The model under review builds one solid part; all positions refer to its coordinate system, in mm. Face numbers are marked on the shaded views. A direction names the side the tool comes from. Give positions to 0.01 mm unless a question says otherwise; leave off trailing zeros. Order: outer loops, then holes, each group sorted by start corner. A loop starts at its lowest first (then second) coordinate and runs counter-clockwise, first axis right, second up. Notation, with made-up numbers: (-19.75, 85) - (38.25, 85) arc R17 cw to (38.25, 99) - close; hole circle Ø6 at (-38.5, 12.5). An arc over 180 degrees is marked (long way). Use a Markdown table: item, result. Add a question column.
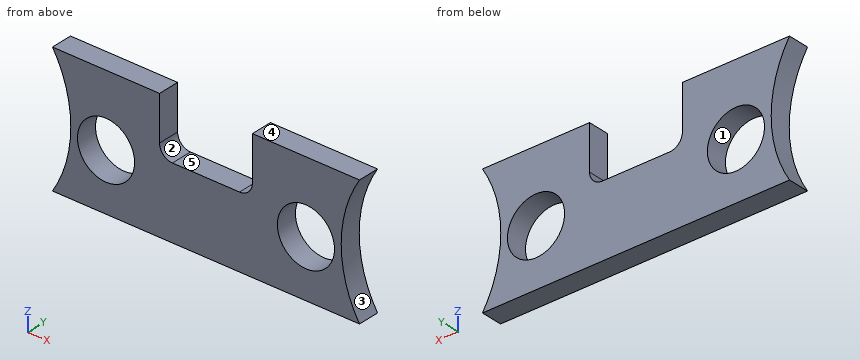
```python
from build123d import *

# Parameters (mm, degrees)
F0_W     = 273.05
F0_H     = 114.3
F1_DEPTH = 19.05
F2_R     = 25.4
F3_DEPTH = 25.4
F5_DEPTH = 25.4
F7_DEPTH = 25.4


with BuildPart() as f1:
    # F0 (on Front) → F1 (new body)
    with BuildSketch(Plane.XZ):
        with Locations((136.525, 57.15)):
            Rectangle(F0_W, F0_H)
    extrude(amount=F1_DEPTH)

    # F2 (on face) → F3 (cut)
    with BuildSketch(Plane.XZ.offset(19.05)):
        with Locations((47.625, 50.8)):
            Circle(F2_R)
        with Locations((225.425, 50.8)):
            Circle(F2_R)
    extrude(amount=-F3_DEPTH, mode=Mode.SUBTRACT)

    # F4 (on face) → F5 (cut)
    with BuildSketch(Plane.XZ.offset(19.05)):
        with BuildLine():
            Line((177.8, 114.3), (95.25, 114.3))
            Line((95.25, 114.3), (95.25, 74.93))
            ThreePointArc((95.25, 74.93), (98.597769, 66.847769), (106.68, 63.5))
            Line((106.68, 63.5), (166.37, 63.5))
            ThreePointArc((166.37, 63.5), (174.452231, 66.847769), (177.8, 74.93))
            Line((177.8, 74.93), (177.8, 114.3))
        make_face()
    extrude(amount=-F5_DEPTH, mode=Mode.SUBTRACT)

    # F6 (on face) → F7 (cut)
    with BuildSketch(Plane.XZ.offset(19.05)):
        with BuildLine():
            Line((0, 114.3), (0, 0))
            ThreePointArc((0, 0), (16.273098, 57.15), (0, 114.3))
        make_face()
        with BuildLine():
            ThreePointArc((273.05, 114.3), (256.776902, 57.15), (273.05, 0))
            Line((273.05, 0), (273.05, 114.3))
        make_face()
    extrude(amount=-F7_DEPTH, mode=Mode.SUBTRACT)


solid = f1.part
```
Q1. Wall thickness on probe 1 along X at (y, z) = (-2.5, 48); probe 2 along X at (y, z) = (-9.25, 62); probe 3 along Z at (x, y) = (161, -14): over which ranges is each line inside the solid? List them lowest first.
Q2. We need section B-B (z = 93). Write out the cut boundary in (x, y), plus the area to 3 significant figures.
Q3. Draft analysis for pull direction X (two halves, no side actions). For the marked faces 3, 4 and 5, state which applies: pulls with the +X half, pulls with the -X half, needs draft (parallel to the pull), parting line crosses it, or undercut.
Q4. Machinability: for the marked faces 1 and 2, which of the approach directions +Z, -Z, +X, -X, +Y, -Y give a long, thin tool a straight path to every point of the face, cutting with its end or side? Answer none if there is none.
Q5. We need section C-C (x = 31). Write out the cut boundary in (y, z), plus the area to 3 significant figures.
Q6. Clearance check with flat-ended pins moving along their axes: P1, Ø6, axis at x = 114, y = -9.5, coming from the +Z side; P2, Ø2, axis at y = -13, z = 55.5, coming from the -X side; P3, Ø2, axis at y = -8.5, z = 91.5, coming from the -X side. State where each tip first meets the part, or that it passes through.
Q7. We need section D-D (z = 50.8). Write out the cut boundary in (x, y) (3 decimals), plus the area to 3 significant figures.
Q8. We need section A-A (y = -10.5). Write out the cut boundary in (x, z) (3 decimals).
Here are the results:
| question | item | result |
|---|---|---|
| 1 | probe 1 | 15.89 to 22.38, 72.87 to 200.18, 250.67 to 257.16 |
| 1 | probe 2 | 16.16 to 24.83, 70.42 to 202.63, 248.22 to 256.89 |
| 1 | probe 3 | 0 to 63.5 |
| 2 | outline | (10.18, -19.05) - (95.25, -19.05) - (95.25, 0) - (10.18, 0) - close; (177.8, -19.05) - (262.87, -19.05) - (262.87, 0) - (177.8, 0) - close |
| 2 | area | 3,240 mm2 |
| 3 | face 3 | pulls with the +X half |
| 3 | face 4 | needs draft |
| 3 | face 5 | undercut |
| 4 | face 1 | +Y, -Y |
| 4 | face 2 | +Z, +Y, -Y |
| 5 | outline | (-19.05, 0) - (0, 0) - (0, 31.6) - (-19.05, 31.6) - close; (-19.05, 70) - (0, 70) - (0, 114.3) - (-19.05, 114.3) - close |
| 5 | area | 1,450 mm2 |
| 6 | P1 | z = 63.5 |
| 6 | P2 | x = 16.24 |
| 6 | P3 | x = 10.35 |
| 7 | outline | (16.087, -19.05) - (22.225, -19.05) - (22.225, 0) - (16.087, 0) - close; (73.025, -19.05) - (200.025, -19.05) - (200.025, 0) - (73.025, 0) - close; (250.825, -19.05) - (256.963, -19.05) - (256.963, 0) - (250.825, 0) - close |
| 7 | area | 2,650 mm2 |
| 8 | outline | (0, 0) - (273.05, 0) arc R108.49 cw to (273.05, 114.3) - (177.8, 114.3) - (177.8, 74.93) arc R11.43 cw to (166.37, 63.5) - (106.68, 63.5) arc R11.43 cw to (95.25, 74.93) - (95.25, 114.3) - (0, 114.3) arc R108.49 cw to start; hole circle Ø50.8 at (47.625, 50.8); hole circle Ø50.8 at (225.425, 50.8) |
